Part model, mm, in its own coordinate system. Round coordinates to 2 decimals unless told otherwise and drop trailing zeros. Loops run counter-clockwise (first coordinate to the right, second up) from the corner with the lowest first, then second, coordinate; pieces in that order, holes last. Notation, with made-up numbers: M -14.75,-13.75 L -7.75,-13.75 A9 cw -7.75,-2.75 Z; hole C 3.25,57 d1. An arc over 180 degrees is marked long. Answer as CSV lines item,"result". Start each with the question number.
Item 1: Band-saw the part on A-A (y = 0). Give the cut face in (x, z) (3 decimals).
Item 2: Band-saw the part on D-D (z = -2.05). Give the cut face in (x, y) (3 decimals).
Item 3: Drop flat-ended pins along their axis: pin 1 Ø1.5 at (x, y) = (-4.5, -0.5) entering from +Z; pin 2 Ø1.2 at (y, z) = (0, 0) entering from +X (3 decimals). Give the stop position or say it passes through.
Item 4: Wall check: line 1 (Y direction, x = -15, z = 0); line 2 (Y direction, x = -8.5, z = 0.1). Give the ranges that are in metal, low to high.
Item 5: Band-saw the part on C-C (x = -8.5). Give the cut face in (y, z), and give its area (3 significant figures).
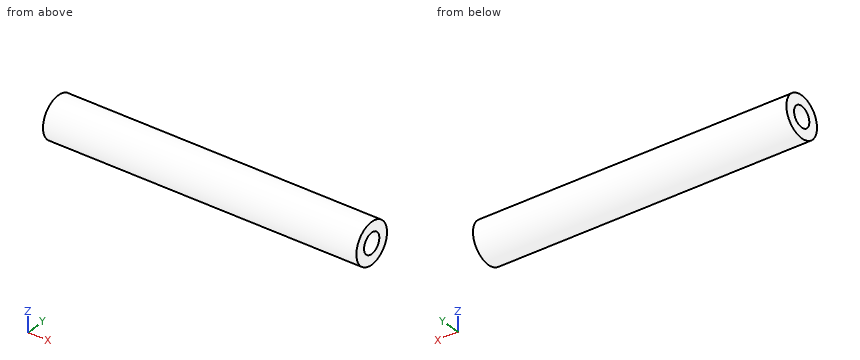
```python
from build123d import *

# Parameters (mm, degrees)
SCHIZZO2_R                   = 2.51
SCHIZZO2_R_2                 = 1
ESTRUSIONE_ESTRUSIONE1_DEPTH = 19.125


with BuildPart() as part:
    # Schizzo2 → Estrusione-Estrusione1 (new, symmetric)
    with BuildSketch(Plane(origin=(0, 0, 0), x_dir=(0, 0, -1), z_dir=(1, 0, 0))):
        Circle(SCHIZZO2_R)
        Circle(SCHIZZO2_R_2, mode=Mode.SUBTRACT)
    extrude(amount=ESTRUSIONE_ESTRUSIONE1_DEPTH, both=True)

    # Schizzo5 → Foro filettato M3x0.5-2 (revolve, cut)
    with BuildSketch(Plane(origin=(19.125, 0, 0), x_dir=(0, 0, -1), z_dir=(0, 1, 0))):
        Polygon((0, 0), (0, 8.751075774), (1.25, 8), (1.25, 0), align=None)
    foro_filettato_m3x0_5_2 = revolve(axis=Axis((25.475, 0, 0), (-1, 0, 0)), mode=Mode.SUBTRACT)

    # Specchia1: Foro filettato M3x0.5-2 across plane
    add(foro_filettato_m3x0_5_2.mirror(Plane(origin=(0, 0, 0), x_dir=(0, 0, 1), z_dir=(1, 0, 0))), mode=Mode.SUBTRACT)


solid = part.part
```
Answer block:
1,outline,"M -19.125,-2.51 L 19.125,-2.51 L 19.125,-1.25 L 11.125,-1.25 L 10.975,-1 L -10.975,-1 L -11.125,-1.25 L -19.125,-1.25 Z; M -19.125,1.25 L -11.125,1.25 L -10.975,1 L 10.975,1 L 11.125,1.25 L 19.125,1.25 L 19.125,2.51 L -19.125,2.51 Z"
2,outline,"M -19.125,-1.448 L 19.125,-1.448 L 19.125,1.448 L -19.125,1.448 Z"
3,pin 1,"stops at z = 2.51"
3,pin 2,"passes through"
4,line 1,"y = -2.51 to -1.25, 1.25 to 2.51"
4,line 2,"y = -2.51 to -0.99, 0.99 to 2.51"
5,outline,"C 0,0 d5.02; hole C 0,0 d2"
5,area,"16.7 mm^2"
